Geometry: final body of the model. Coordinates: model frame, mm. Round coordinates to 2 decimals unless told otherwise and drop trailing zeros. Loops run counter-clockwise (first coordinate to the right, second up) from the corner with the lowest first, then second, coordinate; pieces in that order, holes last. Notation, with made-up numbers: M -39.75,4 L -5.75,4 A28 ccw -5.75,33 Z; hole C 17,-7 d6. An arc over 180 degrees is marked long. Return JSON: item names as keys, results as strings.
from build123d import *

# Parameters (mm, degrees)
PAD002_DEPTH = 0.4
SKETCH005_W  = 14
SKETCH005_H  = 13
PAD003_DEPTH = 1
FILLET_R     = 0.5


with BuildPart() as part:
    # Sketch004 → Pad002 (new body)
    with BuildSketch(Plane.XY):
        with BuildLine():
            Line((-8.25, 7.75), (-8.25, -7.75))
            ThreePointArc((-8.25, -7.75), (-8.103553, -8.103553), (-7.75, -8.25))
            Line((-7.75, -8.25), (7.75, -8.25))
            ThreePointArc((7.75, -8.25), (8.103553, -8.103553), (8.25, -7.75))
            Line((8.25, -7.75), (8.25, 7.75))
            ThreePointArc((8.25, 7.75), (8.103553, 8.103553), (7.75, 8.25))
            Line((7.75, 8.25), (-7.75, 8.25))
            ThreePointArc((-7.75, 8.25), (-8.103553, 8.103553), (-8.25, 7.75))
        make_face()
    extrude(amount=PAD002_DEPTH)

    # Sketch005 (on Face10 of Pad002) → Pad003 (join)
    with BuildSketch(Plane.XY.offset(0.4)):
        Rectangle(SKETCH005_W, SKETCH005_H)
    extrude(amount=PAD003_DEPTH)

    # Fillet
    fillet_edges = [part.edges().sort_by_distance(p)[0] for p in [
        (-7, 0, 1.4),
        (0, -6.5, 1.4),
        (7, 0, 1.4),
        (0, 6.5, 1.4),
    ]]
    fillet(fillet_edges, radius=FILLET_R)


solid = part.part
Q1. Section query B-B (x = 6). Output: boundary loops of the cut face in (y, z).
Determined:
{"outline": "M -8.25,0 L 8.25,0 L 8.25,0.4 L 6.5,0.4 L 6.5,0.9 A0.5 ccw 6,1.4 L -6,1.4 A0.5 ccw -6.5,0.9 L -6.5,0.4 L -8.25,0.4 Z"}
Q2. Section query C-C (z = 0.7). Output: boundary loops of the cut face in (x, y).
Determined:
{"outline": "M -7,-6.5 L 7,-6.5 L 7,6.5 L -7,6.5 Z"}
Q3. Material intervals for L1, parallel to X at y = -5, z = 0.9; L2, parallel to Y at x = -2.75, z = 0.6; L3, parallel to Z at x = 7.75, y = 2, sorted ascending.
Determined:
{"L1": "x = -7 to 7", "L2": "y = -6.5 to 6.5", "L3": "z = 0 to 0.4"}
Q4. Section query A-A (y = 2.5). Output: boundary loops of the cut face in (x, z), plus the area to 3 significant figures.
Determined:
{"outline": "M -8.25,0 L 8.25,0 L 8.25,0.4 L 7,0.4 L 7,0.9 A0.5 ccw 6.5,1.4 L -6.5,1.4 A0.5 ccw -7,0.9 L -7,0.4 L -8.25,0.4 Z", "area": "20.5 mm^2"}
